Here's how the part is built. I have some questions about the finished solid (model axes, mm). Face numbers are marked on the shaded views. Round coordinates to 2 decimals unless told otherwise and drop trailing zeros. Loops run counter-clockwise (first coordinate to the right, second up) from the corner with the lowest first, then second, coordinate; pieces in that order, holes last. Notation, with made-up numbers: (47, -36) - (97, -36) arc R23 cw to (97, -9) - close; hole circle Ø8 at (-40, -36). An arc over 180 degrees is marked (long way). Return JSON: item names as keys, results as strings. Group by question number.
```python
from build123d import *

# Parameters (mm, degrees)
SKETCH1_R           = 2.4
BOSS_EXTRUDE1_DEPTH = 56.59882


with BuildPart() as part:
    # Sketch1 → Boss-Extrude1 (new body)
    with BuildSketch(Plane.XY):
        with BuildLine():
            Line((-76.173191063, 182.117156823), (-79.348191063, 182.096951811))
            Line((-79.348191063, 182.096951811), (-79.348191063, 204.196458108))
            ThreePointArc((-79.348191063, 204.196458108), (-81.394050197, 209.135598974), (-86.333191063, 211.181458108))
            Line((-86.333191063, 211.181458108), (-92.778191065, 211.181458108))
            Line((-92.778191065, 211.181458108), (-92.778191065, 208.926458108))
            ThreePointArc((-92.778191065, 208.926458108), (-98.778191065, 202.926458108), (-104.778191065, 208.926458108))
            Line((-104.778191065, 208.926458108), (-104.778191065, 214.356458108))
            Line((-104.778191065, 214.356458108), (-92.778191065, 214.356458108))
            Line((-92.778191065, 214.356458108), (-86.333191063, 214.356458108))
            ThreePointArc((-86.333191063, 214.356458108), (-79.148986166, 211.380663005), (-76.173191063, 204.196458108))
            Line((-76.173191063, 204.196458108), (-76.173191063, 182.117156823))
        make_face()
        with Locations((-98.778191065, 208.926458108)):
            Circle(SKETCH1_R, mode=Mode.SUBTRACT)
    extrude(amount=BOSS_EXTRUDE1_DEPTH)


solid = part.part
```
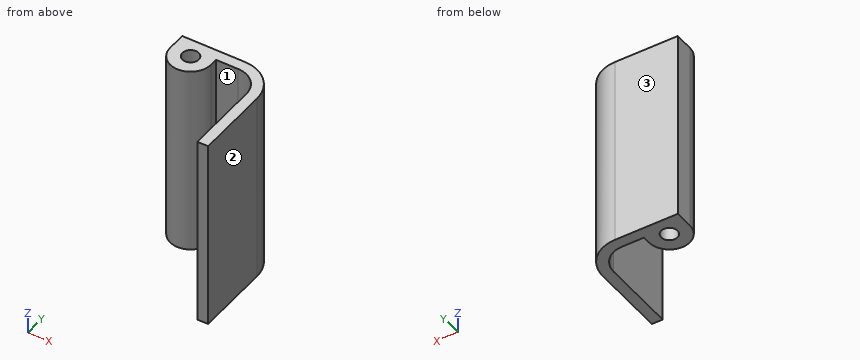
Q1. Will these pins go through, and if not, where does the flat tip stop? pin 1 Ø1 at (y, z) = (193, 45.5) entering from -X; pin 2 Ø3 at (x, z) = (-101.5, 27) entering from -Y; pin 3 Ø1.8 at (y, z) = (209.5, 36) entering from +X.
Q2. If we mould it in two halves opening along X, with no side actions, what happens to the marked faces 1, 2 and 3? For each: +X half, -X half, draft (parallel to the pull), parting line (faces both ways), or undercut.
Q3. Imagine slicing it at C-C, the plane y = 208. List the corners of the cut face in (x, z) for me, and give its area (3 significant figures).
Q4. Imagine slicing it at B-B, the plane x = -99. List the corners of the cut face in (y, z) for me.
Q5. Imagine slicing it at D-D, the plane y = 198. List the corners of the cut face in (x, z) for me, and give its area (3 significant figures).
Q6. Please list where these lines run through material, in increasing order: line 1 (X direction, y = 189.5, z = 19); line 2 (Y direction, x = -97, z = 54.5); line 3 (X direction, y = 205, z = 19).
Q7. Imagine slicing it at A-A, the plane z = 50. List the corners of the cut face in (x, y) for me (3 decimals).
Output values:
{
 "1": {"pin 1": "stops at x = -79.35", "pin 2": "stops at y = 203.05", "pin 3": "stops at x = -77.18"},
 "2": {"face 1": "undercut", "face 2": "+X half", "face 3": "draft"},
 "3": {"outline": "(-104.71, 0) - (-100.99, 0) - (-100.99, 56.6) - (-104.71, 56.6) - close; (-96.56, 0) - (-92.85, 0) - (-92.85, 56.6) - (-96.56, 56.6) - close; (-80.47, 0) - (-76.91, 0) - (-76.91, 56.6) - (-80.47, 56.6) - close", "area": "622 mm^2"},
 "4": {"outline": "(202.93, 0) - (206.54, 0) - (206.54, 56.6) - (202.93, 56.6) - close; (211.32, 0) - (214.36, 0) - (214.36, 56.6) - (211.32, 56.6) - close"},
 "5": {"outline": "(-79.35, 0) - (-76.17, 0) - (-76.17, 56.6) - (-79.35, 56.6) - close", "area": "180 mm^2"},
 "6": {"line 1": "x = -79.35 to -76.17", "line 2": "y = 203.2 to 207.31, 210.54 to 214.36", "line 3": "x = -103.32 to -94.24, -79.39 to -76.21"},
 "7": {"outline": "(-104.778, 208.926) arc R6 ccw to (-92.778, 208.926) - (-92.778, 211.181) - (-86.333, 211.181) arc R6.985 cw to (-79.348, 204.196) - (-79.348, 182.097) - (-76.173, 182.117) - (-76.173, 204.196) arc R10.16 ccw to (-86.333, 214.356) - (-104.778, 214.356) - close; hole circle Ø4.8 at (-98.778, 208.926)"}
}
